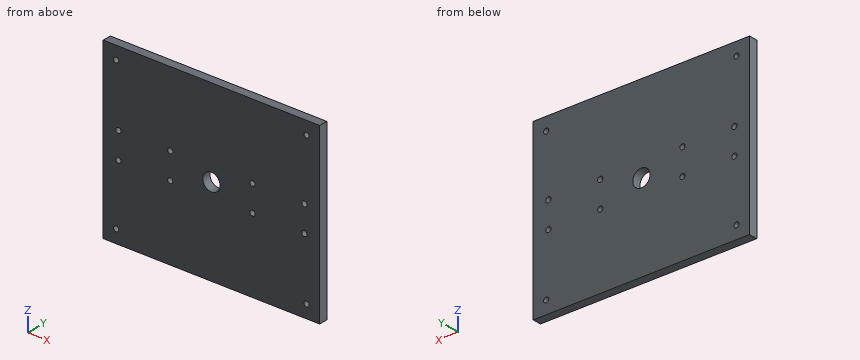
from build123d import *

# Parameters (mm, degrees)
SKETCH1_W                = 100
SKETCH1_H                = 80
BOSS_EXTRUDE1_DEPTH      = 4
M2_CLEARANCE_HOLE1_D     = 2.4
M2_CLEARANCE_HOLE1_DEPTH = 6
M2_CLEARANCE_HOLE2_D     = 2.4
M2_CLEARANCE_HOLE2_DEPTH = 6
F_8_0MM_DOWEL_HOLE1_D    = 8


with BuildPart() as part:
    # Sketch1 → Boss-Extrude1 (new body)
    with BuildSketch(Plane(origin=(0, 0, 0), x_dir=(1, 0, 0), z_dir=(0, 1, 0))):
        with Locations((50, 40)):
            Rectangle(SKETCH1_W, SKETCH1_H)
    extrude(amount=BOSS_EXTRUDE1_DEPTH)

    # M2 Clearance Hole1
    with Locations(Plane(origin=(0, 4, 0), x_dir=(1, 0, 0), z_dir=(0, 1, 0))):
        with Locations((7, 34), (31, 34), (31, 46), (7, 46)):
            m2_clearance_hole1 = Hole(M2_CLEARANCE_HOLE1_D / 2, depth=M2_CLEARANCE_HOLE1_DEPTH)

    # Mirror1: M2 Clearance Hole1 across plane
    add(m2_clearance_hole1.mirror(Plane.ZY.offset(-50)), mode=Mode.SUBTRACT)

    # M2 Clearance Hole2
    with Locations(Plane(origin=(0, 4, 0), x_dir=(1, 0, 0), z_dir=(0, 1, 0))):
        with Locations((6, 74), (94, 74), (94, 6), (6, 6)):
            Hole(M2_CLEARANCE_HOLE2_D / 2, depth=M2_CLEARANCE_HOLE2_DEPTH)

    # Ø8.0mm Dowel Hole1 (through all)
    with Locations(Plane(origin=(0, 4, 0), x_dir=(1, 0, 0), z_dir=(0, 1, 0))):
        with Locations((50, 40)):
            Hole(F_8_0MM_DOWEL_HOLE1_D / 2)


solid = part.part
Here's how the part is built. I have some questions about the finished solid (model axes, mm). Coordinates: 2 decimals unless noted, no trailing zeros. Order: outer loops, then holes, each group sorted by start corner. A loop starts at its lowest first (then second) coordinate and runs counter-clockwise, first axis right, second up. Notation, with made-up numbers: M 34.5,32.25 L 77.5,32.25 A18 cw 77.5,44.25 Z; hole C 25.5,84 d8. An arc over 180 degrees is marked long. Answer as CSV lines item,"result".
Item 1: Imagine slicing it at A-A on x = 50. Write out the boundary of the cut face in (y, z).
Results found:
outline,"M 0,-80 L 4,-80 L 4,-44 L 0,-44 Z; M 0,-36 L 4,-36 L 4,0 L 0,0 Z"
Item 2: Imagine slicing it at D-D on z = -6. Write out the boundary of the cut face in (x, y), plus the area to 3 significant figures.
Results found:
outline,"M 0,0 L 4.8,0 L 4.8,4 L 0,4 Z; M 7.2,0 L 92.8,0 L 92.8,4 L 7.2,4 Z; M 95.2,0 L 100,0 L 100,4 L 95.2,4 Z"
area,"381 mm2"
Item 3: Imagine slicing it at B-B on z = -40. Write out the boundary of the cut face in (x, y), plus the area to 3 significant figures.
Results found:
outline,"M 0,0 L 46,0 L 46,4 L 0,4 Z; M 54,0 L 100,0 L 100,4 L 54,4 Z"
area,"368 mm2"
Item 4: If I drill on line 1 (X direction, y = 2.5, z = -74); line 2 (Z direction, x = 31, y = 2.8); line 3 (Z direction, x = 93, y = 3), over which ranges is the centre line in solid material (lowest first)?
Results found:
line 1,"0 to 4.8, 7.2 to 92.8, 95.2 to 100"
line 2,"-80 to -47.2, -44.8 to -35.2, -32.8 to 0"
line 3,"-80 to -74.66, -73.34 to -47.2, -44.8 to -35.2, -32.8 to -6.66, -5.34 to 0"
Item 5: Imagine slicing it at C-C on x = 31. Write out the boundary of the cut face in (y, z).
Results found:
outline,"M 0,-80 L 4,-80 L 4,-47.2 L 0,-47.2 Z; M 0,-44.8 L 4,-44.8 L 4,-35.2 L 0,-35.2 Z; M 0,-32.8 L 4,-32.8 L 4,0 L 0,0 Z"
Item 6: For pin 1 (3 mm diameter, centred on x = 6, z = -74, fed in from -Y), with a flat end and sliding along its axis, tell me the tip position at first contact or that it passes through.
Results found:
pin 1,"y = 0"
